Design review of the part built by this model. Coordinates are the model's own, in mm. Round coordinates to 2 decimals unless told otherwise and drop trailing zeros. Write each loop counter-clockwise with the first axis right and the second up, starting at its lowest first coordinate (ties: lowest second). Pieces come first, ordered by that corner, then holes. Notation, with made-up numbers: (-7.75, -11.5) - (22.25, -11.5) arc R24 ccw to (22.25, 19.5) - close; hole circle Ø5 at (59.25, 11). An arc over 180 degrees is marked (long way). Use one line per item in the form item = value.
```python
from build123d import *

# Parameters (mm, degrees)
F0_W     = 6
F0_H     = 120
F1_DEPTH = 20
F2_R     = 2.1
F3_DEPTH = 20
F4_R     = 2.75
F5_DEPTH = 25


with BuildPart() as f1:
    # F0 (on Top) → F1 (new body)
    with BuildSketch(Plane.XY):
        with Locations((3, -60)):
            Rectangle(F0_W, F0_H)
    extrude(amount=F1_DEPTH)

    # F2 (on face) → F3 (cut)
    with BuildSketch(Plane.XY.offset(20)):
        with Locations((3, -14)):
            Circle(F2_R)
        with Locations((3, -106)):
            Circle(F2_R)
        with Locations((3, -60)):
            Circle(F2_R)
    extrude(amount=-F3_DEPTH, mode=Mode.SUBTRACT)

    # F4 (on face) → F5 (cut)
    with BuildSketch(Plane.YZ.offset(6)):
        with Locations((-115, 15)):
            Circle(F4_R)
        with Locations((-115, 5)):
            Circle(F4_R)
        with Locations((-5, 5)):
            Circle(F4_R)
        with Locations((-5, 15)):
            Circle(F4_R)
    extrude(amount=-F5_DEPTH, mode=Mode.SUBTRACT)


solid = f1.part
```
Q1. We need section B-B on y = -106. Write out the cut boundary in (x, z), then the cut area to 3 significant figures.
Calculated:
outline = (0, 0) - (0.9, 0) - (0.9, 20) - (0, 20) - close; (5.1, 0) - (6, 0) - (6, 20) - (5.1, 20) - close
area = 36.0 mm2
Q2. We need section A-A on z = 15. Write out the cut boundary in (x, y).
Calculated:
outline = (0, -120) - (6, -120) - (6, -117.75) - (0, -117.75) - close; (0, -112.25) - (6, -112.25) - (6, -7.75) - (0, -7.75) - close; (0, -2.25) - (6, -2.25) - (6, 0) - (0, 0) - close; hole circle Ø4.2 at (3, -106); hole circle Ø4.2 at (3, -60); hole circle Ø4.2 at (3, -14)
Q3. To check wall thickness, follow line 1 along Z through (x, y) = (1.9, -115); line 2 along Y through (x, z) = (3, 13.75); line 3 along Z through (x, y) = (3.05, -6.5). State the ranges of each line that lie inside material, in increasing order. Write a range as from..to.
Calculated:
line_1 = 0..2.25, 7.75..12.25, 17.75..20
line_2 = -120..-117.45, -112.55..-108.1, -103.9..-62.1, -57.9..-16.1, -11.9..-7.45, -2.55..0
line_3 = 0..2.7, 7.3..12.7, 17.3..20
Q4. Draft analysis for pull direction Y (two halves, no side actions). For faces 1 (the cylindrical face through (3.042, -117.747, 15.121)), 2 (the flat face through (0.3, -59.2, 20)), 3 (the cylindrical face through (2.54, -108.05, 10.14)), 4 (the flat face through (3, -120, 10)), state which applies: released by +Y, released by -Y, zero draft, split by the parting line, or undercut.
Calculated:
face_1 = undercut
face_2 = zero draft
face_3 = undercut
face_4 = released by -Y
Q5. We need section C-C on x = 2.8. Write out the cut boundary in (y, z), then the cut area to 3 significant figures.
Calculated:
outline = (-120, 0) - (-108.09, 0) - (-108.09, 20) - (-120, 20) - close; (-103.91, 0) - (-62.09, 0) - (-62.09, 20) - (-103.91, 20) - close; (-57.91, 0) - (-16.09, 0) - (-16.09, 20) - (-57.91, 20) - close; (-11.91, 0) - (0, 0) - (0, 20) - (-11.91, 20) - close; hole circle Ø5.5 at (-115, 5); hole circle Ø5.5 at (-115, 15); hole circle Ø5.5 at (-5, 5); hole circle Ø5.5 at (-5, 15)
area = 2,050 mm2
Q6. For P1, Ø3, axis at x = 2, z = 11.5, coming from the +Y side; P2, Ø5, axis at y = -115, z = 15, coming from the -X side, all flat-tipped, find the tip position at first contact; note any pin that passes through.
Calculated:
P1 = 0
P2 = through
Q7. We need section D-D on y = -5. Write out the cut boundary in (x, z), then the cut area to 3 significant figures.
Calculated:
outline = (0, 0) - (6, 0) - (6, 2.25) - (0, 2.25) - close; (0, 7.75) - (6, 7.75) - (6, 12.25) - (0, 12.25) - close; (0, 17.75) - (6, 17.75) - (6, 20) - (0, 20) - close
area = 54.0 mm2
